The model under review builds one solid part; all positions refer to its coordinate system, in mm. Round coordinates to 2 decimals unless told otherwise and drop trailing zeros. Write each loop counter-clockwise with the first axis right and the second up, starting at its lowest first coordinate (ties: lowest second). Pieces come first, ordered by that corner, then holes. Notation, with made-up numbers: (79.25, 75) -> (129.25, 75) arc R17 cw to (129.25, 85) -> close; hole circle Ø6 at (-4.5, 12.25). An arc over 180 degrees is marked (long way). Use CSV: the item, a comma, the result in double quotes. Start each with the question number.
1) For pin 1 Ø5 at (x, z) = (-56, -3) entering from +Y; pin 2 Ø1.5 at (x, y) = (10.5, -4.5) entering from -Z; pin 3 Ø5 at (y, z) = (-23, -3.5) entering from -X, all flat-tipped, find the tip position at first contact; note any pin that passes through.
2) Take a section at A-A, the plane y = 22. Give the boundary of the cut face in (x, z), then the cut area to 3 significant figures.
3) Take a section at B-B, the plane x = 55.5. Give the boundary of the cut face in (y, z).
4) Wall thickness on probe 1 along Z at (x, y) = (-50.5, 19); probe 2 along Z at (x, y) = (22.5, 23): over which ranges is each line inside the solid? List them lowest first. Write a range as [from, to].
5) Take a section at C-C, the plane y = 11.5. Give the boundary of the cut face in (x, z).
from build123d import *

# Parameters (mm, degrees)
SKETCH_1_W      = 150
SKETCH_1_H      = 65
EXTRUDE_1_DEPTH = 95
SKETCH_2_W      = 1
SKETCH_2_H      = 7


with BuildPart() as part:
    # 草图1 → 拉伸1 (new body)
    with BuildSketch(Plane.XY):
        Rectangle(SKETCH_1_W, SKETCH_1_H)
    extrude(amount=EXTRUDE_1_DEPTH)

    # 扫描1: sweep along a path in 草图3
    with BuildLine(Plane(origin=(0, 19, 0), x_dir=(-1, 0, 0), z_dir=(0, 1, 0))) as sweep_1_path:
        Line((59.5, 0), (59.5, -4))
        Line((59.5, -4), (48.5, -4))
    # 草图2 → 扫描1 (sweep)
    with BuildSketch(Plane(origin=(0, 0, 0), x_dir=(-1, 0, 0), z_dir=(0, 0, -1))):
        with Locations((59.5, 22)):
            Rectangle(SKETCH_2_W, SKETCH_2_H)
    sweep_1 = sweep(path=sweep_1_path.line, transition=Transition.RIGHT)

    # 镜向1: 扫描1 across plane
    add(sweep_1.mirror(Plane.ZX))


solid = part.part
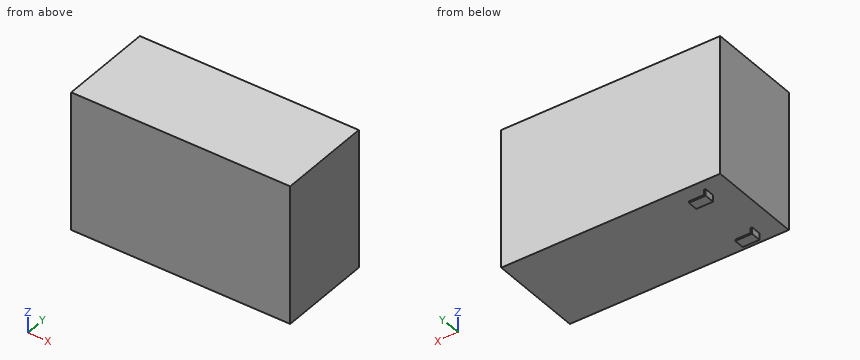
Values found:
1,pin 1,"y = 25.5"
1,pin 2,"z = 0"
1,pin 3,"x = -60"
2,outline,"(-75, 0) -> (-60, 0) -> (-60, -4.5) -> (-48.5, -4.5) -> (-48.5, -3.5) -> (-59, -3.5) -> (-59, 0) -> (75, 0) -> (75, 95) -> (-75, 95) -> close"
2,area,"14,300 mm²"
3,outline,"(-32.5, 0) -> (32.5, 0) -> (32.5, 95) -> (-32.5, 95) -> close"
4,probe 1,"[-4.5, -3.5], [0, 95]"
4,probe 2,"[0, 95]"
5,outline,"(-75, 0) -> (75, 0) -> (75, 95) -> (-75, 95) -> close"
